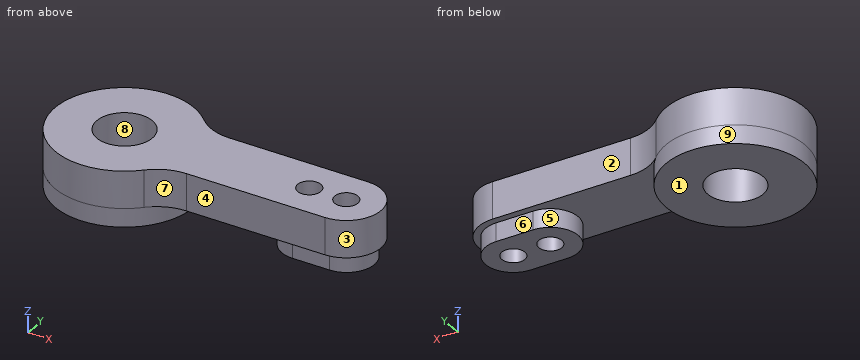
```python
from build123d import *

# Parameters (mm, degrees)
SKETCH_R      = 3
SKETCH_R_2    = 1.25
PAD_DEPTH     = 4
SKETCH001_R   = 7.5
SKETCH001_R_2 = 3
PAD001_DEPTH  = 2
SKETCH002_R   = 1.25
PAD002_DEPTH  = 2


with BuildPart() as part:
    # Sketch → Pad (new body)
    with BuildSketch(Plane.XY):
        with BuildLine():
            Line((9, 3.750318), (23.96134, 3.750318))
            ThreePointArc((23.96134, -3.749682), (27.71134, 0.000318), (23.96134, 3.750318))
            Line((9, -3.749682), (23.96134, -3.749682))
            ThreePointArc((9, -3.749682), (7.034594, -4.137023), (5.36312, -5.241118))
            ThreePointArc((5.338537, 5.266156), (-7.498804, -0.017545), (5.36312, -5.241118))
            ThreePointArc((5.338537, 5.266156), (7.018581, 4.144257), (9, 3.750318))
        make_face()
        Circle(SKETCH_R, mode=Mode.SUBTRACT)
        with Locations((23.96134, 0.000318)):
            Circle(SKETCH_R_2, mode=Mode.SUBTRACT)
        with Locations((19.96134, 0)):
            Circle(SKETCH_R_2, mode=Mode.SUBTRACT)
    extrude(amount=PAD_DEPTH)

    # Sketch001 (on Face10 of Pad) → Pad001 (join)
    with BuildSketch(Plane(origin=(0, 0, 0), x_dir=(1, 0, 0), z_dir=(0, 0, -1))):
        Circle(SKETCH001_R)
        Circle(SKETCH001_R_2, mode=Mode.SUBTRACT)
    extrude(amount=PAD001_DEPTH)

    # Sketch002 (on Face5 of Pad001) → Pad002 (join)
    with BuildSketch(Plane(origin=(0, 0, 0), x_dir=(1, 0, 0), z_dir=(0, 0, -1))):
        with BuildLine():
            ThreePointArc((20, 3), (17, 0), (20, -3))
            Line((20, -3), (24, -3))
            ThreePointArc((24, -3), (27, 0), (24, 3))
            Line((20, 3), (24, 3))
        make_face()
        with Locations((20, 0)):
            Circle(SKETCH002_R, mode=Mode.SUBTRACT)
        with Locations((24, 0)):
            Circle(SKETCH002_R, mode=Mode.SUBTRACT)
    extrude(amount=PAD002_DEPTH)


solid = part.part
```
Here's how the part is built. I have some questions about the finished solid (model axes, mm). Face numbers are marked on the shaded views. A direction names the side the tool comes from. Coordinates: 2 decimals unless noted, no trailing zeros. Loops run counter-clockwise (first coordinate to the right, second up) from the corner with the lowest first, then second, coordinate; pieces in that order, holes last. Notation, with made-up numbers: (61, -1.5) - (84, -1.5) arc R11 cw to (84, 10.5) - close; hole circle Ø8 at (-5.5, 79.5). An arc over 180 degrees is marked (long way). Return JSON: item names as keys, results as strings. Group by question number.
Item 1: Will these pins go through, and if not, where does the flat tip stop? P1, Ø3, axis at x = 19.96, y = 0, coming from the +Z side; P2, Ø1.6, axis at x = 22, z = -1, coming from the -Y side; P3, Ø2, axis at x = 13, z = 2.5, coming from the -Y side; P4, Ø1, axis at x = 23.5, y = 0, coming from the +Z side.
Item 2: On a 3-axis mill with a long thin cutter (end or side, diameter ignored), from which of +Z, -Z, +X, -X, +Y, -Y can I reach the whole of each face in a straight line? I mean the marked faces 1, 2, 3, 4 and 5. Say none if no direction works.
Item 3: If we section it at A-A on z = -0.6: Write out the boundary of the cut face in (x, y), and give its area (3 significant figures).
Item 4: We'd pull the mould along X, two halves only. Please class the marked faces 6, 7, 8 and 9: +X half, -X half, draft (parallel to the pull), parting line (faces both ways), or undercut.
Item 5: If we section it at B-B on z = 1.75: Write out the boundary of the cut face in (x, y).
Item 6: I need wall thicknesses on line 1 (X direction, y = 0, z = -0.5); line 2 (Y direction, x = 20, z = -1.15); line 3 (X direction, y = -0.5, z = 2.45). Which ranges of each line are inside material? Lowest first, please. Write a range as from..to.
Calculated:
{
 "1": {"P1": "stops at z = 4", "P2": "stops at y = -3", "P3": "stops at y = -3.75", "P4": "passes through"},
 "2": {"face 1": "-Z, +X, -X, +Y, -Y", "face 2": "+Z, -Z, +X, +Y", "face 3": "+Z, -Z, +X", "face 4": "+Z, -Z, +X, -Y", "face 5": "-Z"},
 "3": {"outline": "circle Ø15 at (0, 0); (20, -3) - (24, -3) arc R3 ccw to (24, 3) - (20, 3) arc R3 ccw to start; hole circle Ø6 at (0, 0); hole circle Ø2.5 at (20, 0); hole circle Ø2.5 at (24, 0)", "area": "191 mm^2"},
 "4": {"face 6": "draft", "face 7": "+X half", "face 8": "undercut", "face 9": "undercut"},
 "5": {"outline": "(5.34, 5.27) arc R7.5 ccw (long way) to (5.36, -5.24) arc R5.18 cw to (9, -3.75) - (23.96, -3.75) arc R3.75 ccw to (23.96, 3.75) - (9, 3.75) arc R5.18 cw to start; hole circle Ø6 at (0, 0); hole circle Ø2.5 at (19.96, 0); hole circle Ø2.5 at (23.96, 0)"},
 "6": {"line 1": "x = -7.5..-3, 3..7.5, 17..18.75, 21.25..22.75, 25.25..27", "line 2": "y = -3..-1.25, 1.25..3", "line 3": "x = -7.48..-2.96, 2.96..18.82, 21.11..22.82, 25.11..27.68"}
}
